Here's how the part is built. I have some questions about the finished solid (model axes, mm). Round coordinates to 2 decimals unless told otherwise and drop trailing zeros. Write each loop counter-clockwise with the first axis right and the second up, starting at its lowest first coordinate (ties: lowest second). Pieces come first, ordered by that corner, then holes. Notation, with made-up numbers: (18.25, 86) -> (31.25, 86) arc R9 ccw to (31.25, 92) -> close; hole circle Ø8 at (-2.75, 30). An arc over 180 degrees is marked (long way). Answer in a Markdown table with one row per item.
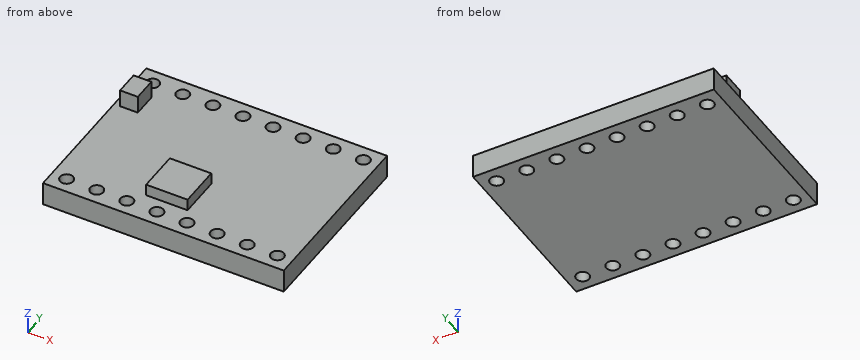
from build123d import *

# Parameters (mm, degrees)
F0_W     = 20.32
F0_H     = 15.24
F0_R     = 0.55
F1_DEPTH = 2
F3_W     = 1.5
F3_H     = 2
F4_DEPTH = 1.5
F3_W_2   = 3.5
F3_H_2   = 3.5
F5_DEPTH = 1


with BuildPart() as f1:
    # F0 (on Top) → F1 (new body)
    with BuildSketch(Plane.XY):
        with Locations((10.16, 7.62)):
            Rectangle(F0_W, F0_H)
        with Locations((1.27, 1.27)):
            Circle(F0_R, mode=Mode.SUBTRACT)
        with Locations((3.81, 1.27)):
            Circle(F0_R, mode=Mode.SUBTRACT)
        with Locations((6.35, 1.27)):
            Circle(F0_R, mode=Mode.SUBTRACT)
        with Locations((8.89, 1.27)):
            Circle(F0_R, mode=Mode.SUBTRACT)
        with Locations((11.43, 1.27)):
            Circle(F0_R, mode=Mode.SUBTRACT)
        with Locations((13.97, 1.27)):
            Circle(F0_R, mode=Mode.SUBTRACT)
        with Locations((16.51, 1.27)):
            Circle(F0_R, mode=Mode.SUBTRACT)
        with Locations((19.05, 1.27)):
            Circle(F0_R, mode=Mode.SUBTRACT)
        with Locations((1.27, 13.97)):
            Circle(F0_R, mode=Mode.SUBTRACT)
        with Locations((3.81, 13.97)):
            Circle(F0_R, mode=Mode.SUBTRACT)
        with Locations((6.35, 13.97)):
            Circle(F0_R, mode=Mode.SUBTRACT)
        with Locations((8.89, 13.97)):
            Circle(F0_R, mode=Mode.SUBTRACT)
        with Locations((11.43, 13.97)):
            Circle(F0_R, mode=Mode.SUBTRACT)
        with Locations((13.97, 13.97)):
            Circle(F0_R, mode=Mode.SUBTRACT)
        with Locations((16.51, 13.97)):
            Circle(F0_R, mode=Mode.SUBTRACT)
        with Locations((19.05, 13.97)):
            Circle(F0_R, mode=Mode.SUBTRACT)
    extrude(amount=F1_DEPTH)

    # F3 (on offset) → F4 (join)
    with BuildSketch(Plane.XY.offset(2)):
        with Locations((1.25, 11.5)):
            Rectangle(F3_W, F3_H)
    extrude(amount=F4_DEPTH)

    # F3 (on offset) → F5 (join)
    with BuildSketch(Plane.XY.offset(2)):
        with Locations((9, 4.29)):
            Rectangle(F3_W_2, F3_H_2)
    extrude(amount=F5_DEPTH)


solid = f1.part
1) I want a section at A-A, the plane x = 1.27. List the corners of the cut face in (y, z) for me.
Response:
| item | result |
|---|---|
| outline | (0, 0) -> (0.72, 0) -> (0.72, 2) -> (0, 2) -> close; (1.82, 0) -> (13.42, 0) -> (13.42, 2) -> (12.5, 2) -> (12.5, 3.5) -> (10.5, 3.5) -> (10.5, 2) -> (1.82, 2) -> close; (14.52, 0) -> (15.24, 0) -> (15.24, 2) -> (14.52, 2) -> close |
2) I want a section at C-C, the plane z = 1.35. Count the separate pieces of the cut face and the enclosed holes in it, and give its area (3 significant figures).
Response:
| item | result |
|---|---|
| separate pieces | 1 |
| enclosed holes | 16 |
| area | 294 mm^2 |
3) I want a section at D-D, the plane x = 19.05. List the corners of the cut face in (y, z) for me.
Response:
| item | result |
|---|---|
| outline | (0, 0) -> (0.72, 0) -> (0.72, 2) -> (0, 2) -> close; (1.82, 0) -> (13.42, 0) -> (13.42, 2) -> (1.82, 2) -> close; (14.52, 0) -> (15.24, 0) -> (15.24, 2) -> (14.52, 2) -> close |
4) I need wall thicknesses on line 1 (Y direction, x = 16.51, z = 1.25); line 2 (Y direction, x = 6, z = 1.8); line 3 (Z direction, x = 2.5, y = 11.75). Which ranges of each line are inside material? Lowest first, please. Write a range as [from, to].
Response:
| item | result |
|---|---|
| line 1 | y = [0, 0.72], [1.82, 13.42], [14.52, 15.24] |
| line 2 | y = [0, 0.85], [1.69, 13.55], [14.39, 15.24] |
| line 3 | z = [0, 2] |
5) I want a section at B-B, the plane z = 2.65. List the corners of the cut face in (x, y) for me.
Response:
| item | result |
|---|---|
| outline | (0.5, 10.5) -> (2, 10.5) -> (2, 12.5) -> (0.5, 12.5) -> close; (7.25, 2.54) -> (10.75, 2.54) -> (10.75, 6.04) -> (7.25, 6.04) -> close |
6) For pin 1 (0.8 mm diameter, centred on y = 5, z = 2.5, fed in from -X); pin 2 (1.3 mm diameter, centred on x = 19.05, y = 13.97, fed in from -Z); pin 3 (1.8 mm diameter, centred on x = 1.27, y = 13.97, fed in from +Z); pin 4 (1 mm diameter, centred on x = 8.5, y = 4.5, fed in from +Z), each with a flat end and sliding along its axis, tell me the tip position at first contact or that it passes through.
Response:
| item | result |
|---|---|
| pin 1 | stops at x = 7.25 |
| pin 2 | stops at z = 0 |
| pin 3 | stops at z = 2 |
| pin 4 | stops at z = 3 |
